```python
from build123d import *

# Parameters (mm, degrees)
EXTRUDE_1_DEPTH = 82
FILLET_1_R      = 3


with BuildPart() as part:
    # 草图1 → 凸台-拉伸1 (new body)
    with BuildSketch(Plane.XY):
        Polygon((0, 0), (0, 2), (3, 2), (13, 12), (13, 37), (3, 47), (-54, 47), (-54, 49), (3, 49), (15, 37), (15, 12), (3, 0), align=None)
    extrude(amount=EXTRUDE_1_DEPTH)

    # 圆角1
    fillet_1_edges = [part.edges().sort_by_distance(p)[0] for p in [
        (3, 2, 41),
        (13, 12, 41),
        (13, 37, 41),
        (3, 47, 41),
        (3, 49, 41),
        (15, 37, 41),
        (15, 12, 41),
        (3, 0, 41),
    ]]
    fillet(fillet_1_edges, radius=FILLET_1_R)


solid = part.part
```
CAD build for the part. Positions are in the model's coordinates, mm. A direction names the side the tool comes from. Coordinates: 2 decimals unless noted, no trailing zeros. Order: outer loops, then holes, each group sorted by start corner. A loop starts at its lowest first (then second) coordinate and runs counter-clockwise, first axis right, second up. Notation, with made-up numbers: (38.25, 81) - (96.25, 81) arc R28 cw to (96.25, 109) - close; hole circle Ø5 at (18, 80). An arc over 180 degrees is marked (long way). Answer in a Markdown table with one row per item.
1. Pull direction Y, two halves, no side cores. Call faces 1 (the face through (2.921, 0.235, 41.574)), 2 (the face through (-54, 48, 40)), 3 (the face through (2.89, 48.78, 41.57)), 4 (the face through (2.89, 2.22, 41.57)): +Y half, -Y half, draft (parallel to the pull), parting line (faces both ways), or undercut.
Answer:
| item | result |
|---|---|
| face 1 | -Y half |
| face 2 | draft |
| face 3 | +Y half |
| face 4 | undercut |
2. Slice it at A-A, the plane z = 50.5. List the corners of the cut face in (x, y).
Answer:
| item | result |
|---|---|
| outline | (-54, 47) - (1.76, 47) arc R3 cw to (3.88, 46.12) - (12.12, 37.88) arc R3 cw to (13, 35.76) - (13, 13.24) arc R3 cw to (12.12, 11.12) - (3.88, 2.88) arc R3 cw to (1.76, 2) - (0, 2) - (0, 0) - (1.76, 0) arc R3 ccw to (3.88, 0.88) - (14.12, 11.12) arc R3 ccw to (15, 13.24) - (15, 35.76) arc R3 ccw to (14.12, 37.88) - (3.88, 48.12) arc R3 ccw to (1.76, 49) - (-54, 49) - close |
3. Flat gauge pins, fed straight in: P1, Ø4, axis at y = 8, z = 54, coming from the +X side; P2, Ø18, axis at y = 24.5, z = 28.5, coming from the -X side; P3, Ø1.6, axis at y = 0.5, z = 30, coming from the -X side. Where does each tip first touch, or does it go through?
Answer:
| item | result |
|---|---|
| P1 | x = 13 |
| P2 | x = 13 |
| P3 | x = 0 |
4. Slice it at C-C, the plane y = 18. List the corners of the cut face in (x, z).
Answer:
| item | result |
|---|---|
| outline | (13, 0) - (15, 0) - (15, 82) - (13, 82) - close |
5. 3-axis set-ups, long thin cutter, end or side, ignore diameter. For faces 5 (the face through (0, 1, 40)), 6 (the face through (9, 43, 40)), 7 (the face through (8, 7, 40)): which of +Z, -Z, +X, -X, +Y, -Y reach the whole face in a straight line?
Answer:
| item | result |
|---|---|
| face 5 | +Z, -Z, -X, -Y |
| face 6 | +Z, -Z, +X, +Y |
| face 7 | +Z, -Z, -X |
6. Slice it at B-B, the plane x = -20. List the corners of the cut face in (y, z), then the cut area to 3 significant figures.
Answer:
| item | result |
|---|---|
| outline | (47, 0) - (49, 0) - (49, 82) - (47, 82) - close |
| area | 164 mm² |
7. Drill centre lines: L1, parallel to Y at x = -11, z = 37.5; L2, parallel to X at y = 30.5, z = 17; L3, parallel to X at y = 39.5, z = 70. Where is each one in solid material? Low to high. Write a range as from..to.
Answer:
| item | result |
|---|---|
| L1 | 47..49 |
| L2 | 13..15 |
| L3 | 10.5..12.5 |
